from build123d import *

# Parameters (mm, degrees)
SKETCH2_R           = 101.6
BOSS_EXTRUDE1_DEPTH = 76.2
FILLET1_R           = 10.16
CUT_EXTRUDE1_REACH  = 164.639
SKETCH3_R           = 6.35
CUT_EXTRUDE2_REACH  = 164.639


with BuildPart() as part:
    # Sketch2 → Boss-Extrude1 (new body)
    with BuildSketch(Plane.XY):
        Circle(SKETCH2_R)
    extrude(amount=-BOSS_EXTRUDE1_DEPTH)

    # Fillet1
    fillet1_edges = [part.edges().sort_by_distance(p)[0] for p in [
        (-101.6, 0, 0),
        (-101.6, 0, -76.2),
    ]]
    fillet(fillet1_edges, radius=FILLET1_R)

    # Sketch3 → Cut-Extrude1 (cut, up to next)
    with BuildSketch(Plane.XY, mode=Mode.PRIVATE) as cut_extrude1_sk1:
        Circle(SKETCH3_R)
    cut_extrude1_tool1 = extrude(cut_extrude1_sk1.sketch, amount=-CUT_EXTRUDE1_REACH, mode=Mode.PRIVATE) & part.part
    add(cut_extrude1_tool1.solids().sort_by_distance((0, 0, 0))[0], mode=Mode.SUBTRACT)

    # Sketch5 → Cut-Extrude2 (cut, up to next)
    with BuildSketch(Plane.XY, mode=Mode.PRIVATE) as cut_extrude2_sk1:
        with BuildLine():
            Line((65.773312704, 63.522790682), (25.453227454, 28.350365292))
            ThreePointArc((25.453227454, 28.350365292), (32.796836191, 19.390140171), (37.108086442, 8.637124558))
            Line((37.108086442, 8.637124558), (86.518715929, 29.593671518))
            ThreePointArc((86.518715929, 29.593671518), (78.012894947, 47.699704631), (65.773312704, 63.522790682))
        make_face()
    cut_extrude2_tool1 = extrude(cut_extrude2_sk1.sketch, amount=-CUT_EXTRUDE2_REACH, mode=Mode.PRIVATE) & part.part
    # Sketch5 → Cut-Extrude2 (cut, up to next)
    with BuildSketch(Plane.XY, mode=Mode.PRIVATE) as cut_extrude2_sk2:
        with BuildLine():
            Line((63.522790682, -65.773312704), (28.350365292, -25.453227454))
            ThreePointArc((28.350365292, -25.453227454), (19.390140171, -32.796836191), (8.637124558, -37.108086442))
            Line((8.637124558, -37.108086442), (29.593671518, -86.518715929))
            ThreePointArc((29.593671518, -86.518715929), (47.699704631, -78.012894947), (63.522790682, -65.773312704))
        make_face()
    cut_extrude2_tool2 = extrude(cut_extrude2_sk2.sketch, amount=-CUT_EXTRUDE2_REACH, mode=Mode.PRIVATE) & part.part
    # Sketch5 → Cut-Extrude2 (cut, up to next)
    with BuildSketch(Plane.XY, mode=Mode.PRIVATE) as cut_extrude2_sk3:
        with BuildLine():
            Line((-65.773312704, -63.522790682), (-25.453227454, -28.350365292))
            ThreePointArc((-25.453227454, -28.350365292), (-32.796836191, -19.390140171), (-37.108086442, -8.637124558))
            Line((-37.108086442, -8.637124558), (-86.518715929, -29.593671518))
            ThreePointArc((-86.518715929, -29.593671518), (-78.012894947, -47.699704631), (-65.773312704, -63.522790682))
        make_face()
    cut_extrude2_tool3 = extrude(cut_extrude2_sk3.sketch, amount=-CUT_EXTRUDE2_REACH, mode=Mode.PRIVATE) & part.part
    # Sketch5 → Cut-Extrude2 (cut, up to next)
    with BuildSketch(Plane.XY, mode=Mode.PRIVATE) as cut_extrude2_sk4:
        with BuildLine():
            Line((-63.522790682, 65.773312704), (-28.350365292, 25.453227454))
            ThreePointArc((-28.350365292, 25.453227454), (-19.390140171, 32.796836191), (-8.637124558, 37.108086442))
            Line((-8.637124558, 37.108086442), (-29.593671518, 86.518715929))
            ThreePointArc((-29.593671518, 86.518715929), (-47.699704631, 78.012894947), (-63.522790682, 65.773312704))
        make_face()
    cut_extrude2_tool4 = extrude(cut_extrude2_sk4.sketch, amount=-CUT_EXTRUDE2_REACH, mode=Mode.PRIVATE) & part.part
    add(cut_extrude2_tool1.solids().sort_by_distance((56.84773, 34.461957, 0))[0], mode=Mode.SUBTRACT)
    add(cut_extrude2_tool2.solids().sort_by_distance((34.461957, -56.84773, 0))[0], mode=Mode.SUBTRACT)
    add(cut_extrude2_tool3.solids().sort_by_distance((-56.84773, -34.461957, 0))[0], mode=Mode.SUBTRACT)
    add(cut_extrude2_tool4.solids().sort_by_distance((-34.461957, 56.84773, 0))[0], mode=Mode.SUBTRACT)


solid = part.part
Could you check a few things on this model? Use its own coordinates, in mm. A direction names the side the tool comes from. Give positions to 0.01 mm unless a question says otherwise; leave off trailing zeros. Order: outer loops, then holes, each group sorted by start corner. A loop starts at its lowest first (then second) coordinate and runs counter-clockwise, first axis right, second up.
1. For faces 1 (the flat face through (19, 1, -76.2)), 2 (the cylindrical face through (47.46, -78.16, -37.57)), which set-ups out of +Z, -Z, +X, -X, +Y, -Y let a thin tool reach every point of the face, with its end or its side?
2. Suppose I cut it at A-A (x = 0). List the corners of the cut face in (y, z) for me, plus the area to 3 significant figures.
3. I need wall thicknesses on L1, parallel to Y at x = 0, z = -48; L2, parallel to X at y = -47.5, z = -8.5; L3, parallel to Y at x = -50, z = -60. Which ranges of each line are inside material? Lowest first, please.
4. Will these pins go through, and if not, where does the flat tip stop? P1, Ø2, axis at y = -27.5, z = -64, coming from the -X side; P2, Ø8, axis at x = -55.5, z = -30.5, coming from the -Y side; P3, Ø8, axis at x = 28, z = -18, coming from the +Y side.
5. Suppose I cut it at D-D (z = -6). List the corners of the cut face in (x, y) for me.
6. Suppose I cut it at B-B (z = -35.5). List the corners of the cut face in (x, y) for me.
7. We'd pull the mould along X, two halves only. Please class faces 3 (the flat face through (19, 1, 0)), 4 (the cylindrical face through (-22.025, -99.184, -37.709)), 5 (the cylindrical face through (-47.46, 78.16, -37.57)): pulls with the +X half, pulls with the -X half, needs draft (parallel to the pull), parting line crosses it, or undercut.
Solved:
1. face 1: -Z, +X, -X, +Y, -Y
1. face 2: +Z, -Z
2. outline: (-101.6, -66.04) arc R10.16 ccw to (-91.44, -76.2) - (-6.35, -76.2) - (-6.35, 0) - (-91.44, 0) arc R10.16 ccw to (-101.6, -10.16) - close; (6.35, -76.2) - (91.44, -76.2) arc R10.16 ccw to (101.6, -66.04) - (101.6, -10.16) arc R10.16 ccw to (91.44, 0) - (6.35, 0) - close
2. area: 14,400 mm2
3. L1: y = -101.6 to -6.35, 6.35 to 101.6
3. L2: x = -89.66 to -78.13, -47.41 to 13.04, 47.58 to 89.66
3. L3: y = -88.45 to -49.76, -14.1 to 50.27, 76.56 to 88.45
4. P1: stops at x = -98.08
4. P2: stops at y = -87.58
4. P3: stops at y = 98.72
5. outline: circle Ø201.42 at (0, 0); hole (-86.52, -29.59) arc R91.44 ccw to (-65.77, -63.52) - (-25.45, -28.35) arc R38.1 cw to (-37.11, -8.64) - close; hole (-63.52, 65.77) - (-28.35, 25.45) arc R38.1 cw to (-8.64, 37.11) - (-29.59, 86.52) arc R91.44 ccw to start; hole circle Ø12.7 at (0, 0); hole (8.64, -37.11) - (29.59, -86.52) arc R91.44 ccw to (63.52, -65.77) - (28.35, -25.45) arc R38.1 cw to start; hole (25.45, 28.35) arc R38.1 cw to (37.11, 8.64) - (86.52, 29.59) arc R91.44 ccw to (65.77, 63.52) - close
6. outline: circle Ø203.2 at (0, 0); hole (-86.52, -29.59) arc R91.44 ccw to (-65.77, -63.52) - (-25.45, -28.35) arc R38.1 cw to (-37.11, -8.64) - close; hole (-63.52, 65.77) - (-28.35, 25.45) arc R38.1 cw to (-8.64, 37.11) - (-29.59, 86.52) arc R91.44 ccw to start; hole circle Ø12.7 at (0, 0); hole (8.64, -37.11) - (29.59, -86.52) arc R91.44 ccw to (63.52, -65.77) - (28.35, -25.45) arc R38.1 cw to start; hole (25.45, 28.35) arc R38.1 cw to (37.11, 8.64) - (86.52, 29.59) arc R91.44 ccw to (65.77, 63.52) - close
7. face 3: needs draft
7. face 4: parting line crosses it
7. face 5: undercut
